Autodesk Inventor part; units mm, degrees
ref_plane "YZ Plane" through (0, 0, 0) normal (1, 0, 0) x (0, 1, 0)
ref_plane "XZ Plane" through (0, 0, 0) normal (0, 1, 0) x (-1, 0, 0)
ref_plane "XY Plane" through (0, 0, 0) normal (0, 0, 1) x (1, 0, 0)
sketch "Szkic1" plane through (0, 0, 0) normal (0, 1, 0) x (-1, 0, 0)
  line L0 (-3.66, 66.34) -> (-3.66, 0)
  line L1 (-3.66, 0) -> (3.66, 0) construction
  line L2 (3.66, 0) -> (3.66, 66.34)
  arc A0 (-3.66, 0) -> (3.66, 0) centre (0, 0) ccw
  circle A1 centre (0, 0) radius 2.55
  line L3 (3.66, 12) -> (-3.66, 12)
  line L4 (3.66, 66.34) -> (-3.66, 66.34)
  line L5 (3.66, 56.34) -> (-3.66, 56.34)
  line L6 (0, 66.34) -> (0, 75) construction
  line L7 (-3.66, 52) -> (-7.16, 52)
  line L8 (-7.16, 52) -> (-7.16, 50.4)
  line L9 (-7.16, 50.4) -> (-3.66, 50.4)
  line L10 (-3.66, 50.4) -> (-3.66, 52)
  arc A2 (-7.16, 57.6) -> (-7.16, 50.4) centre (-7.16, 54) ccw
  arc A3 (-7.16, 56) -> (-7.16, 52) centre (-7.16, 54) ccw
  line L11 (-7.16, 57.6) -> (-5.46, 57.6)
  line L12 (-5.46, 57.6) -> (-5.46, 56)
  line L13 (-5.46, 56) -> (-7.16, 56)
  point P0 (0, -3.66)
  point P1 (0, 12)
  dimension "d0" = 7.32
  dimension "d3" = 5.1
  dimension "d17" = 12
  dimension "d26" = 70
  dimension "d27" = 60
  dimension "d30" = 75
  dimension "d31" = 8.66
  dimension "d35" = 2
  dimension "d36" = 3.6
  dimension "d37" = 3.5
  dimension "d38" = 1.7
  dimension "d39" = 52
extrude "Wyciągnięcie proste1" add sketch "Szkic1" along normal mid plane 24 contours L5 L2 L3 L0 | L2 A0 L0 L3
extrude "Wyciągnięcie proste4" cut sketch "Szkic1" along normal mid plane 8.35 contours L2 A0 L0 L3
extrude "Wyciągnięcie proste6" add sketch "Szkic1" along normal mid plane 7.8 contours L4 L2 L5 L0
sketch "Szkic4" plane through (-3.66, 3.9, 66.34) normal (0, 0, 1) x (1, 0, 0)
  line L0 (7.32, -7.8) -> (0, -7.8)
  line L1 (0, -7.8) -> (7.32, -7.8)
  line L2 (7.32, -7.8) -> (7.32, 0)
  line L3 (7.32, 0) -> (0, 0)
  line L4 (0, 0) -> (0, -7.8)
  line L5 (2.4334, -7.8) -> (0, -4.9)
  line L6 (0, 0.275) -> (0, -8.075)
  line L7 (0, -2.9) -> (2.4334, 0)
  line L8 (0, -3.9) -> (7.32, -3.9) construction
  point P0 (1.2167, -6.35)
  dimension "d43" = 50
  dimension "d44" = 2
extrude "Wyciągnięcie proste7" add sketch "Szkic4" along normal blind 8.66 contours L0 L5 L4 L7 L3 L2
extrude "Wyciągnięcie proste8" add sketch "Szkic1" along normal mid plane 3 contours L0 L9 L8 L7 | L8 A2 L11 L12 L13 A3
equation "\"d33\" = d31"
properties part number "kredafullv3"
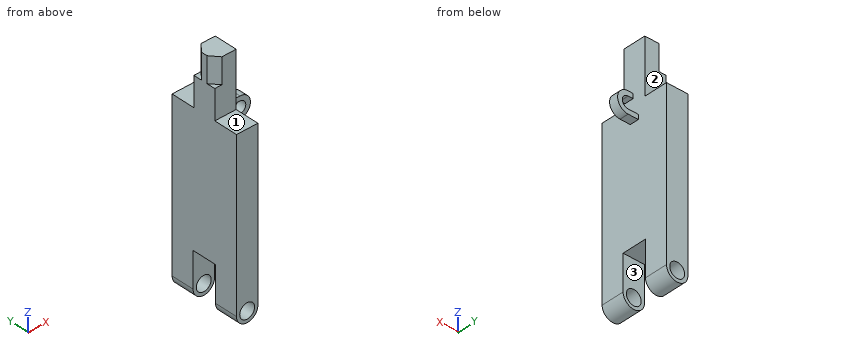
Geometry: final body of the model. Coordinates: model frame, mm. Face numbers are marked on the shaded views. A direction names the side the tool comes from. Round coordinates to 2 decimals unless told otherwise and drop trailing zeros. Write each loop counter-clockwise with the first axis right and the second up, starting at its lowest first coordinate (ties: lowest second). Pieces come first, ordered by that corner, then holes.
Item 1: Section query A-A (x = 0). Return loops of the section in (y, z) (3 decimals), plus the area to 3 significant figures.
Item 2: Section query D-D (z = 14). Return loops of the section in (x, y), plus the area to 3 significant figures.
Item 3: Section query B-B (z = 54). Return loops of the section in (x, y), plus the area to 3 significant figures.
Item 4: Set-up query: the marked faces 1, 2 and 3. Return all of +Z, -Z, +X, -X, +Y, -Y with unobstructed straight access to the full face (end or side cutting, diameter ignored); none if empty.
Item 5: Material intervals for L1, parallel to Z at x = 0, y = 8.25; L2, parallel to Y at x = -1, z = 70.5; L3, parallel to Y at x = 0.5, z = 3.5 (3 decimals), sorted ascending.
Item 6: Section query C-C (y = 10.75). Return loops of the section in (x, z), plus the area to 3 significant figures.
Item 7: Pin query (flat end, axial travel): P1, Ø3, axis at x = 4.5, y = 7.5, coming from the +Z side; P2, Ø4.5, axis at x = 0, z = 0, coming from the +Y side; P3, Ø1.4, axis at x = 6.5, y = -0.5, coming from the +Z side; P4, Ø12, axis at y = -2, z = 46, coming from the +X side. Return the tip coordinate at first contact, or that it passes through.
Completed:
1. outline: (-12, -3.66) - (-4.175, -3.66) - (-4.175, -2.55) - (-12, -2.55) - close; (-12, 2.55) - (-4.175, 2.55) - (-4.175, 12) - (4.175, 12) - (4.175, 2.55) - (12, 2.55) - (12, 56.34) - (3.9, 56.34) - (3.9, 75) - (-3.9, 75) - (-3.9, 56.34) - (-12, 56.34) - close; (4.175, -3.66) - (12, -3.66) - (12, -2.55) - (4.175, -2.55) - close
1. area: 1,370 mm2
2. outline: (-3.66, -12) - (3.66, -12) - (3.66, 12) - (-3.66, 12) - close
2. area: 176 mm2
3. outline: (-3.66, -12) - (3.66, -12) - (3.66, 12) - (-3.66, 12) - close; (9.16, -1.5) - (10.76, -1.5) - (10.76, 1.5) - (9.16, 1.5) - close
3. area: 180 mm2
4. face 1: +Z, +X, -X, -Y
4. face 2: +Z, +X, -X, +Y
4. face 3: -Z, +X, -X
5. L1: z = -3.66 to -2.55, 2.55 to 56.34
5. L2: y = -3.9 to 3.9
5. L3: y = -12 to -4.175, 4.175 to 12
6. outline: (-3.66, 0) arc R3.66 ccw to (3.66, 0) - (3.66, 56.34) - (-3.66, 56.34) - close; hole circle Ø5.1 at (0, 0)
6. area: 413 mm2
7. P1: stops at z = 56.34
7. P2: passes through
7. P3: stops at z = 57.6
7. P4: stops at x = 10.14
